```python
from build123d import *

# Parameters (mm, degrees)
BOSS_EXTRUDE1_DEPTH = 12.3
SKETCH2_W           = 2.2
SKETCH2_H           = 2.17
CUT_EXTRUDE1_DEPTH  = 4.2
CUT_EXTRUDE3_DEPTH  = 0.8
SKETCH5_W           = 3
SKETCH5_H           = 1
BOSS_EXTRUDE2_DEPTH = 0.55
BOSS_EXTRUDE3_DEPTH = 3
SKETCH7_W           = 13.013136742
SKETCH7_H           = 0.83
CUT_EXTRUDE4_DEPTH  = 15.056708453
FILLET1_R           = 2
CUT_EXTRUDE5_DEPTH  = 14.785193345


with BuildPart() as part:
    # Sketch1 → Boss-Extrude1 (new body)
    with BuildSketch(Plane.XY):
        with BuildLine():
            Line((0, 0), (0.299997713, 0.173208719))
            Line((0.299997713, 0.173208719), (0.299997713, 1.781598719))
            Line((0.299997713, 1.781598719), (0.299997713, 6.107458719))
            Line((0.299997713, 6.107458719), (3.299997713, 6.107458719))
            Line((3.299997713, 6.107458719), (3.299997713, 0.646828719))
            Line((3.299997713, 0.646828719), (3.299997713, -0.4))
            Line((3.299997713, -0.4), (0.2, -0.4))
            ThreePointArc((0.2, -0.4), (0.058578644, -0.341421356), (0, -0.2))
            Line((0, -0.2), (0, 0))
        make_face()
    extrude(amount=BOSS_EXTRUDE1_DEPTH)

    # Sketch2 → Cut-Extrude1 (cut)
    with BuildSketch(Plane(origin=(0, 6.107458719, 0), x_dir=(1, 0, 0), z_dir=(0, 1, 0))):
        with Locations((2.199997713, -1.085)):
            Rectangle(SKETCH2_W, SKETCH2_H)
        with Locations((2.199997713, -11.215)):
            Rectangle(SKETCH2_W, SKETCH2_H)
    extrude(amount=-CUT_EXTRUDE1_DEPTH, mode=Mode.SUBTRACT)

    # Sketch4 → Cut-Extrude3 (cut)
    with BuildSketch(Plane.ZY.offset(-0.299997713)):
        with BuildLine():
            Line((10.41158, 6.107458719), (12.3, 6.107458719))
            Line((12.3, 6.107458719), (12.3, 2.215929667))
            ThreePointArc((12.3, 2.215929667), (12.02880398, 4.022129667), (11.23913234, 5.669043272))
            ThreePointArc((11.23913234, 5.669043272), (10.879869522, 5.991150317), (10.41158, 6.107458719))
        make_face()
        with BuildLine():
            Line((1.88842, 6.107458719), (0, 6.107458719))
            Line((0, 6.107458719), (0, 2.215929667))
            ThreePointArc((0, 2.215929667), (0.27119602, 4.022129667), (1.06086766, 5.669043272))
            ThreePointArc((1.06086766, 5.669043272), (1.420130478, 5.991150317), (1.88842, 6.107458719))
        make_face()
    extrude(amount=-CUT_EXTRUDE3_DEPTH, mode=Mode.SUBTRACT)

    # Sketch5 → Boss-Extrude2 (add)
    with BuildSketch(Plane.ZY.offset(-0.299997713)):
        with Locations((6.15, 2.281598719)):
            Rectangle(SKETCH5_W, SKETCH5_H)
    extrude(amount=BOSS_EXTRUDE2_DEPTH)

    # Sketch6 → Boss-Extrude3 (add)
    with BuildSketch(Plane.XY.offset(7.65)):
        Polygon((0.299997713, 2.781598719), (0.299997713, 4.373208719), (-0.250002287, 2.781598719), align=None)
    extrude(amount=-BOSS_EXTRUDE3_DEPTH)

    # Sketch7 → Cut-Extrude4 (cut, through all)
    with BuildSketch(Plane.ZY.offset(-0.299997713)):
        with Locations((5.954326159, 5.69245873)):
            Rectangle(SKETCH7_W, SKETCH7_H)
    extrude(amount=-CUT_EXTRUDE4_DEPTH, mode=Mode.SUBTRACT)

    # Fillet1
    fillet1_edges = [part.edges().sort_by_distance(p)[0] for p in [
        (0.699997713, 5.27745873, 0.816134079),
        (0.699997713, 5.27745873, 11.483865921),
    ]]
    fillet(fillet1_edges, radius=FILLET1_R)

    # Sketch8 → Cut-Extrude5 (cut, through all)
    with BuildSketch(Plane.XY.offset(12.3)):
        Polygon((3.299997713, -0.4), (2.502082924, -0.4), (3.299997713, 5.27745873), align=None)
    extrude(amount=-CUT_EXTRUDE5_DEPTH, mode=Mode.SUBTRACT)


solid = part.part
```
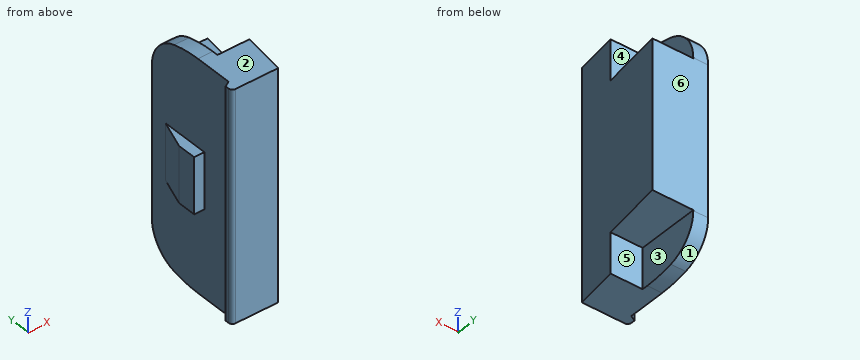
Geometry check sheet. Reference: the model listing, model coordinates, mm. Face numbers are marked on the shaded views. A direction names the side the tool comes from. Give positions to 0.01 mm unless a question says otherwise; leave off trailing zeros. Loops run counter-clockwise (first coordinate to the right, second up) from the corner with the lowest first, then second, coordinate; pieces in that order, holes last. Notation, with made-up numbers: (0, 39.25) - (59, 39.25) arc R23 cw to (59, 75.25) - close; hole circle Ø5 at (8.25, 35). An arc over 180 degrees is marked (long way). Use CSV: the item, a comma, the result in double quotes. Start each with the question number.
Q1. Go/stop test with flat-tipped pins: pin 1 Ø0.5 at (x, z) = (1.5, 1.5) entering from +Y; pin 2 Ø1 at (y, z) = (0.5, 5) entering from +X; pin 3 Ø0.7 at (y, z) = (3.5, 11) entering from +X. Record where each tip stops, or that it passes through.
Q2. Release check for a two-part mould opening along Z. For the marked faces 1, 2 and 3 record: +Z half, -Z half, draft (parallel to the pull), parting line (faces both ways), or undercut.
Q3. Access from +Z, -Z, +X, -X, +Y, -Y to the whole of each face (thin tool, end or side, straight path). Record for the marked faces 4, 5 and 6.
Q4. Scan lines: probe 1 along X at (y, z) = (5, 2); probe 2 along X at (y, z) = (1.6, 7.25); probe 3 along Z at (x, y) = (0.95, 2.4). Record each from-to range of solid material in increasing order. Write a range as from..to.
Q5. Section check B-B, the plane x = 1.55. Record the cut outline in (y, z).
Q6. Section check D-D, the plane x = 0.65. Record the cut outline in (y, z), and give its area (3 significant figures).
Q7. Section check A-A, the plane z = 10. Record the cut outline in (x, y), and give its area (3 significant figures).
Q8. Section check C-C, the plane y = 2.55. Record the cut outline in (x, z).
Findings below:
1,pin 1,"stops at y = 1.91"
1,pin 2,"stops at x = 2.7"
1,pin 3,"stops at x = 1.1"
2,face 1,"-Z half"
2,face 2,"+Z half"
2,face 3,"draft"
3,face 4,"+Z, +X, +Y"
3,face 5,"-Z, +X, +Y"
3,face 6,"+Z, -Z, +X, -X, +Y"
4,probe 1,"x = 0.3..1.1"
4,probe 2,"x = 0.3..2.78"
4,probe 3,"z = 0..12.3"
5,outline,"(-0.4, 0) - (1.91, 0) - (1.91, 2.17) - (5.28, 2.17) - (5.28, 10.13) - (1.91, 10.13) - (1.91, 12.3) - (-0.4, 12.3) - close"
6,outline,"(-0.4, 0) - (2.22, 0) arc R6.15 ccw to (3.79, 0.2) arc R2 ccw to (5.28, 2.14) - (5.28, 10.16) arc R2 ccw to (3.79, 12.1) arc R6.15 ccw to (2.22, 12.3) - (-0.4, 12.3) - close"
6,area,"67.5 mm^2"
7,outline,"(0, -0.2) arc R0.2 ccw to (0.2, -0.4) - (2.5, -0.4) - (3.3, 5.28) - (0.3, 5.28) - (0.3, 0.17) - (0, 0) - close"
7,area,"14.9 mm^2"
8,outline,"(-0.25, 4.65) - (0.3, 4.65) - (0.3, 0.01) - (1.1, 0.01) - (1.1, 2.17) - (2.92, 2.17) - (2.92, 10.13) - (1.1, 10.13) - (1.1, 12.29) - (0.3, 12.29) - (0.3, 7.65) - (-0.25, 7.65) - close"
